Input: part model. Units: mm. Frame: model coordinates. A direction names the side the tool comes from. Round coordinates to 2 decimals unless told otherwise and drop trailing zeros. Answer as CSV lines item,"result". Start each with the question number.
Autodesk Fusion 360 part; units mm, degrees
sketch "Sketch1" plane through (0, 0, 0) normal (0, 0, 1) x (1, 0, 0)
  circle A0 centre (0, 0) radius 3.125
  circle A1 centre (0, 50) radius 3.125
  circle A2 centre (0, 0) radius 13.125
  circle A3 centre (0, 50) radius 13.125
  line L0 (0, 50) -> (0, 0) construction
  line L1 (37.5, 50.1021) -> (37.5, 0.1021) construction
  line L2 (0, 25) -> (18.55, 25) construction
  circle A4 centre (18.55, 25) radius 2.6
  circle A5 centre (18.55, 25) radius 12.6 construction
  line L3 (-10.2863, 8.1521) -> (-1.9703, 18.6453)
  line L4 (-1.8904, 30.9655) -> (-10.3911, 41.9818)
  arc A6 (-1.9703, 18.6453) -> (-1.8904, 30.9655) centre (-9.8074, 24.8564) ccw
  line L5 (75, 25) -> (56.45, 25) construction
  circle A7 centre (56.45, 25) radius 2.6
  circle A8 centre (56.45, 25) radius 12.6 construction
  line L6 (10.6707, 57.6421) -> (15.1766, 51.3504)
  line L7 (50, 25) -> (50, 37.5) construction
  line L8 (0, 0) -> (37.5, 0) construction
  line L9 (18.55, 25) -> (56.45, 25) construction
  line L10 (37.5, 25) -> (37.5, 37.5) construction
  circle A9 centre (50.0503, 50) radius 13.125
  circle A10 centre (50.0503, 50) radius 3.125
  circle A11 centre (50.0503, 0) radius 13.125
  circle A12 centre (50.0503, 0) radius 3.125
  line L11 (29.9485, 49.6973) -> (41.3329, 59.8118)
  line L12 (21.6444, 42.3194) -> (21.6444, 45)
  line L13 (0, 50) -> (50.0503, 50) construction
  arc A13 (15.1766, 51.3504) -> (29.9485, 49.6973) centre (23.3067, 57.173) ccw
  line L14 (63.1753, 50) -> (63.1753, 0)
  line L15 (56.45, 25) -> (61.45, 25) construction
  arc A14 (29.9485, 0.3027) -> (15.1766, -1.3504) centre (23.3067, -7.173) ccw
  line L16 (10.6707, -7.6421) -> (15.1766, -1.3504)
  line L17 (29.9485, 0.3027) -> (41.3329, -9.8118)
  point P0 (5.95, 25)
  dimension "d156" = 6.25
  dimension "d159" = 25
  dimension "d160" = 25
  dimension "d161" = 10
  dimension "d162" = 10
  dimension "d163" = 50
  dimension "d165" = 50
  dimension "d166" = 18.55
  dimension "d167" = 5.2
  dimension "d168" = 10
  dimension "d169" = 10
  dimension "d178" = 37.5
  dimension "d5" = 25
  dimension "d6" = 25
  dimension "d7" = 10
  dimension "d8" = 10
  dimension "d9" = 6.25
  dimension "d10" = 50
  dimension "d11" = 10
  dimension "d12" = 5
extrude "Extrude1" add sketch "Sketch1" along normal blind 12.5
chamfer "Chamfer1" distance 1 angle 45 6 edges at (-2.9135, 51.13, 12.5) (47.1368, 51.13, 12.5) (54.0259, 25.9402, 12.5) (16.1259, 25.9402, 12.5) (47.1368, 1.13, 12.5) (-2.9135, 1.13, 12.5)
fillet "Fillet1" radius 2 14 edges at (12.9237, 54.4962, 12.5) (-7.8314, 60.5326, 12.5) (-6.1408, 36.4737, 12.5) (0.1923, 24.7916, 12.5) (-6.1283, 13.3987, 12.5) (-7.8994, -10.4816, 12.5) (12.9237, -4.4962, 12.5) (22.1945, 2.765, 12.5) (35.6407, -4.7546, 12.5) (55.4285, -11.9725, 12.5) (63.1753, 25, 12.5) (22.1945, 47.235, 12.5) (35.6407, 54.7546, 12.5) (55.4285, 61.9725, 12.5)
sketch "Sketch2" plane through (0, 0, 0) normal (0, 0, -1) x (1, 0, 0)
  circle A0 centre (0, 0) radius 3.125
  line L0 (22.6, -22.6617) -> (18.55, -20.3235)
  line L1 (18.55, -20.3235) -> (14.5, -22.6617)
  line L2 (14.5, -22.6617) -> (14.5, -27.3383)
  line L3 (14.5, -27.3383) -> (18.55, -29.6765)
  line L4 (18.55, -29.6765) -> (22.6, -27.3383)
  line L5 (22.6, -27.3383) -> (22.6, -22.6617)
  circle A1 centre (50.0503, 0) radius 3.125
  circle A2 centre (0, -50) radius 3.125
  circle A3 centre (56.45, -25) radius 2.6
  circle A4 centre (50.0503, -50) radius 3.125
  circle A5 centre (18.55, -25) radius 2.6
  arc A6 (10.6707, 7.6421) -> (-10.2863, -8.1521) centre (0, 0) ccw
  line L6 (-10.2863, -8.1521) -> (-1.9703, -18.6453)
  arc A7 (-1.8904, -30.9655) -> (-1.9703, -18.6453) centre (-9.8074, -24.8564) ccw
  line L7 (-1.8904, -30.9655) -> (-10.3911, -41.9818)
  arc A8 (-10.3911, -41.9818) -> (10.6707, -57.6421) centre (0, -50) ccw
  line L8 (10.6707, -57.6421) -> (15.1766, -51.3504)
  arc A9 (29.9485, -49.6973) -> (15.1766, -51.3504) centre (23.3067, -57.173) ccw
  line L9 (29.9485, -49.6973) -> (41.3329, -59.8118)
  arc A10 (41.3329, -59.8118) -> (63.1753, -50) centre (50.0503, -50) ccw
  line L10 (63.1753, -50) -> (63.1753, 0)
  arc A11 (63.1753, 0) -> (41.3329, 9.8118) centre (50.0503, 0) ccw
  line L11 (41.3329, 9.8118) -> (29.9485, -0.3027)
  arc A12 (15.1766, 1.3504) -> (29.9485, -0.3027) centre (23.3067, 7.173) ccw
  line L12 (15.1766, 1.3504) -> (10.6707, 7.6421)
  point P0 (18.55, -25)
  dimension "d194" = 4.05
extrude "Extrude2" cut sketch "Sketch2" against normal blind 4.5 contours L0 L1 L2 L3 L4 L5
ref_plane "WorkPlane2" through (37.5, 0, 0) normal (1, 0, 0) x (0, 1, 0)
mirror "Mirror5" about plane through (37.5, 0, 0) normal (1, 0, 0) of "Extrude2"
chamfer "Chamfer2" distance 0.5 angle 45 14 edges at (55.4285, -11.9725, 0) (63.1753, 25, 0) (55.4285, 61.9725, 0) (35.6407, 54.7546, 0) (22.1945, 47.235, 0) (12.9237, 54.4962, 0) (-7.8314, 60.5326, 0) (-6.1408, 36.4737, 0) (0.1923, 24.7916, 0) (-6.1283, 13.3987, 0) (-7.8994, -10.4816, 0) (12.9237, -4.4962, 0) (22.1945, 2.765, 0) (35.6407, -4.7546, 0)
equation "d156 = Print6mmOD"
equation "d178 = ( 75 / 2 ) * 1 mm"
equation "d198 = ( 75 / 2 ) * 1 mm"
equation "d9 = Print6mmOD"
equation "Print6mmOD = 6.25 mm"
Item 1: Access query for faces 4 (the face through (-5.75, 36.9, 11.9)), 5 (the face through (54.397, 28.491, 2.218)), 6 (the face through (12.749, -4.305, 0.247)), 7 (the face through (-6.081, 36.397, 5.43)), 8 (the face through (12.89, -4.54, 5.43)). Directions: +Z, -Z, +X, -X, +Y, -Y. A direction counts if a zero-diameter tool reaches every point of the face in a straight line with its end or side. Return the directions, or none.
Item 2: Line query: line 1 (X direction, y = 25, z = 10.25); line 2 (X direction, y = 50.5, z = 9.5); line 3 (Y direction, x = 56.45, z = 7). Output: solid intervals per line, ascending. Write a range as [from, to].
Item 3: Cut plane A-A, the plane y = 25. Give the number of separate pieces and of enclosed holes in the cut face, plus the area to 3 significant figures.
Item 4: Draft query along Y for faces 1 (the face through (16.55, 21.48, 2.22)), 2 (the face through (35.89, 54.64, 0.25)), 3 (the face through (24, 26, 0)). Return one class per face: +Y half, -Y half, draft (parallel to the pull), parting line (faces both ways), or undercut.
Item 5: Pin query (flat end, axial travel): pin 1 Ø7 at (x, y) = (18.55, 25) entering from -Z; pin 2 Ø3.5 at (y, z) = (25, 2.5) entering from -X; pin 3 Ø3 at (x, z) = (54.5, 2) entering from +Y; pin 4 Ø5 at (x, y) = (50.05, 50) entering from -Z. Return the tip coordinate at first contact, or that it passes through.
Results list:
1,face 4,"+Z, -X"
1,face 5,"-Z"
1,face 6,"-Z, -Y"
1,face 7,"+Z, -Z, -X"
1,face 8,"+Z, -Z, -Y"
2,line 1,"[0.19, 15.95], [21.15, 53.85], [59.05, 63.18]"
2,line 2,"[-13.12, -3.08], [3.08, 15.86], [30.85, 46.97], [53.14, 63.17]"
2,line 3,"[-11.46, 22.4], [27.6, 61.46]"
3,separate pieces,"3"
3,enclosed holes,"0"
3,area,"627 mm²"
4,face 1,"undercut"
4,face 2,"+Y half"
4,face 3,"draft"
5,pin 1,"z = 4.5"
5,pin 2,"x = 0.01"
5,pin 3,"y = 62.79"
5,pin 4,"through"
